```python
from build123d import *

# Parameters (mm, degrees)
SKETCH1_R           = 1.45
SKETCH1_W           = 4.5
SKETCH1_H           = 20
BOSS_EXTRUDE1_DEPTH = 5
SKETCH2_W           = 7.5
SKETCH2_H           = 23
SKETCH2_W_2         = 4.5
SKETCH2_H_2         = 20
BOSS_EXTRUDE2_DEPTH = 5
SKETCH3_W           = 7.5
SKETCH3_H           = 23
BOSS_EXTRUDE3_DEPTH = 1
CUT_EXTRUDE1_REACH  = 30.75
SKETCH6_R           = 1.25


with BuildPart() as part:
    # Sketch1 → Boss-Extrude1 (new body)
    with BuildSketch(Plane.XY):
        with BuildLine():
            Line((-4.25, 0), (-4.25, 26))
            ThreePointArc((-4.25, 26), (0, 30.25), (4.25, 26))
            Line((4.25, 26), (4.25, 0))
            ThreePointArc((4.25, 0), (0, -4.25), (-4.25, 0))
        make_face()
        with Locations((0, 26)):
            Circle(SKETCH1_R, mode=Mode.SUBTRACT)
        Circle(SKETCH1_R, mode=Mode.SUBTRACT)
        with Locations((0, 13)):
            Rectangle(SKETCH1_W, SKETCH1_H, mode=Mode.SUBTRACT)
    extrude(amount=BOSS_EXTRUDE1_DEPTH)

    # Sketch2 → Boss-Extrude2 (add)
    with BuildSketch(Plane.XY.offset(5)):
        with Locations((0, 13)):
            Rectangle(SKETCH2_W, SKETCH2_H)
        with Locations((0, 13)):
            Rectangle(SKETCH2_W_2, SKETCH2_H_2, mode=Mode.SUBTRACT)
    extrude(amount=BOSS_EXTRUDE2_DEPTH)

    # Sketch3 → Boss-Extrude3 (add)
    with BuildSketch(Plane.XY.offset(10)):
        with Locations((0, 13)):
            Rectangle(SKETCH3_W, SKETCH3_H)
    extrude(amount=BOSS_EXTRUDE3_DEPTH)

    # Sketch5 → Revolve1 (revolve)
    with BuildSketch(Plane(origin=(0, 0, 0), x_dir=(0, 0, -1), z_dir=(1, 0, 0))):
        with BuildLine():
            Line((-11, 13), (-11, 15.003893641))
            Line((-11, 15.003893641), (-16.924450419, 16.829327494))
            ThreePointArc((-16.924450419, 16.829327494), (-24.885658953, 17.288779267), (-32.151240121, 14.001946821))
            Line((-32.151240121, 14.001946821), (-32.151240121, 13))
            Line((-32.151240121, 13), (-11, 13))
        make_face()
    revolve(axis=Axis((0, 13, 32.151240121), (0, 0, -1)))

    # Sketch6 → Cut-Extrude1 (cut, up to next)
    with BuildSketch(Plane.XZ.offset(-1.5), mode=Mode.PRIVATE) as cut_extrude1_sk1:
        with Locations((0, 7.153891294)):
            Circle(SKETCH6_R)
    cut_extrude1_tool1 = extrude(cut_extrude1_sk1.sketch, amount=-CUT_EXTRUDE1_REACH, mode=Mode.PRIVATE) & part.part
    add(cut_extrude1_tool1.solids().sort_by_distance((0, 1.5, 7.153891))[0], mode=Mode.SUBTRACT)


solid = part.part
```
Geometry: final body of the model. Coordinates: model frame, mm. A direction names the side the tool comes from. Round coordinates to 2 decimals unless told otherwise and drop trailing zeros. Order: outer loops, then holes, each group sorted by start corner. A loop starts at its lowest first (then second) coordinate and runs counter-clockwise, first axis right, second up. Notation, with made-up numbers: (0, -8) -> (22, -8) arc R28 ccw to (22, 14) -> close; hole circle Ø6 at (-36, -31). An arc over 180 degrees is marked (long way). Use one line per item in the form item = value.
(1) Section A-A on y = 24. Return loops of the section in (x, z).
Results list:
outline = (-4.25, 0) -> (4.25, 0) -> (4.25, 5) -> (3.75, 5) -> (3.75, 11) -> (-3.75, 11) -> (-3.75, 5) -> (-4.25, 5) -> close
(2) Draft query along Z for faces 1 (the face through (0.12, 10.276, 13.345)), 2 (the face through (-3, 13, 11)), 3 (the face through (2.25, 13, 5)), 4 (the face through (0, 13, 10)). Return one class per face: pulls with the +Z half, pulls with the -Z half, needs draft (parallel to the pull), parting line crosses it, or undercut.
Results list:
face_1 = undercut
face_2 = undercut
face_3 = needs draft
face_4 = pulls with the -Z half
(3) Access query for faces 5 (the face through (0, 24.5, 8)), 6 (the face through (-3.75, 13, 8)), 7 (the face through (0, 3, 5)), 8 (the face through (0, 1.5, 9)). Directions: +Z, -Z, +X, -X, +Y, -Y. A direction counts if a zero-diameter tool reaches every point of the face in a straight line with its end or side. Return the directions, or none.
Results list:
face_5 = +Z, +X, -X, +Y
face_6 = -X, +Y, -Y
face_7 = -Z
face_8 = +Z, +X, -X, -Y
(4) Ray query, probe 1 along Y at (x, z) = (0, 2.6); probe 2 along Y at (x, z) = (-0.75, 6); probe 3 along Z at (x, y) = (1, 20.5). Return the intervals inside material, ascending. Write a range as [from, to].
Results list:
probe_1 = [-4.25, -1.45], [1.45, 3], [23, 24.55], [27.45, 30.25]
probe_2 = [1.5, 3], [23, 24.5]
probe_3 = [10, 11]
(5) Section B-B on z = 12. Return loops of the section in (x, y), and give its area (3 significant figures).
Results list:
outline = circle Ø4.62 at (0, 13)
area = 16.8 mm^2
(6) First-contact query: pin 1 Ø11 at (y, z) = (14.5, 2.5) entering from +X; pin 2 Ø1.8 at (y, z) = (16, 7) entering from -X; pin 3 Ø5 at (y, z) = (7.5, 21) entering from +X; pin 4 Ø4 at (y, z) = (5.5, 14) entering from -X. Flat tips, straight axial feed; report the tip coordinate or a pass-through.
Results list:
pin_1 = 4.25
pin_2 = -3.75
pin_3 = 3.42
pin_4 = through
